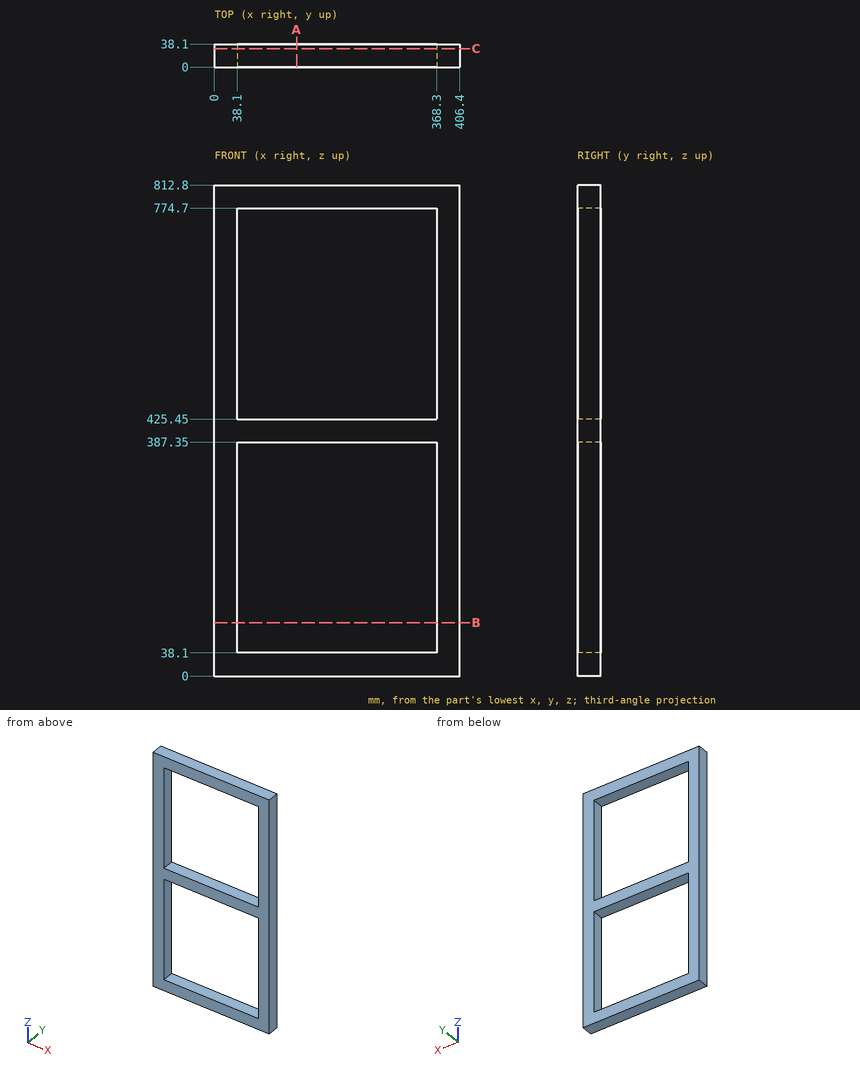
Answer from the drawing. Dimensions are ordinates in mm from the lowest x, y and z of the part. Give positions to 0.01 mm unless a question says otherwise; leave off trailing zeros. Order: outer loops, then holes, each group sorted by start corner. A loop starts at its lowest first (then second) coordinate and runs counter-clockwise, first axis right, second up.
(1) Given pin 1 (1.5 mm diameter, centred on x = 333, z = 427.5, fed in from +Y); pin 2 (11.5 mm diameter, centred on x = 285, y = 21, fed in from -Z), each flat-ended and moving along its own axis, determine where each tip first touches the part or whether it passes through.
(2) Find section B-B (z = 88.5). Give the vertices of the cut face in (x, y).
(3) Find section A-A (x = 136.5). Give the vertices of the cut face in (y, z), plus the area to 3 significant figures.
(4) Straight lines are drawn through the part: L1, parallel to Z at x = 288, y = 6; L2, parallel to X at y = 20, z = 343. For each, find the intervals that lie inside material, in ascending order.
(5) Find section C-C (y = 30.5). Give the vertices of the cut face in (x, z), plus the area to 3 significant figures.
Result sheet:
1. pin 1: passes through
1. pin 2: stops at z = 0
2. outline: (0, 0) - (38.1, 0) - (38.1, 38.1) - (0, 38.1) - close; (368.3, 0) - (406.4, 0) - (406.4, 38.1) - (368.3, 38.1) - close
3. outline: (0, 0) - (38.1, 0) - (38.1, 38.1) - (0, 38.1) - close; (0, 387.35) - (38.1, 387.35) - (38.1, 425.45) - (0, 425.45) - close; (0, 774.7) - (38.1, 774.7) - (38.1, 812.8) - (0, 812.8) - close
3. area: 4,350 mm2
4. L1: z = 0 to 38.1, 387.35 to 425.45, 774.7 to 812.8
4. L2: x = 0 to 38.1, 368.3 to 406.4
5. outline: (0, 0) - (406.4, 0) - (406.4, 812.8) - (0, 812.8) - close; hole (38.1, 38.1) - (368.3, 38.1) - (368.3, 387.35) - (38.1, 387.35) - close; hole (38.1, 425.45) - (368.3, 425.45) - (368.3, 774.7) - (38.1, 774.7) - close
5. area: 99,700 mm2
